Check sheet for the modelled part. Datum: model origin and axes. Units: mm. Give positions to 0.01 mm unless a question says otherwise; leave off trailing zeros. Order: outer loops, then holes, each group sorted by start corner. A loop starts at its lowest first (then second) coordinate and runs counter-clockwise, first axis right, second up.
Item 1: Sectioned sample at C-C on x = 363. Record the boundary of the cut face in (y, z).
Item 2: Sectioned sample at D-D on y = 85. Record the boundary of the cut face in (x, z), and give its area (3 significant figures).
Item 3: Sectioned sample at B-B on z = 16. Record the boundary of the cut face in (x, y), and give its area (3 significant figures).
Item 4: Material ranges on line 1 along Y through (x, z) = (-82, 11.25); line 2 along Y through (x, z) = (64.5, 5.25), recorded low to high.
Item 5: Sectioned sample at A-A on y = 49.5. Record the boundary of the cut face in (x, z), and give its area (3 significant figures).
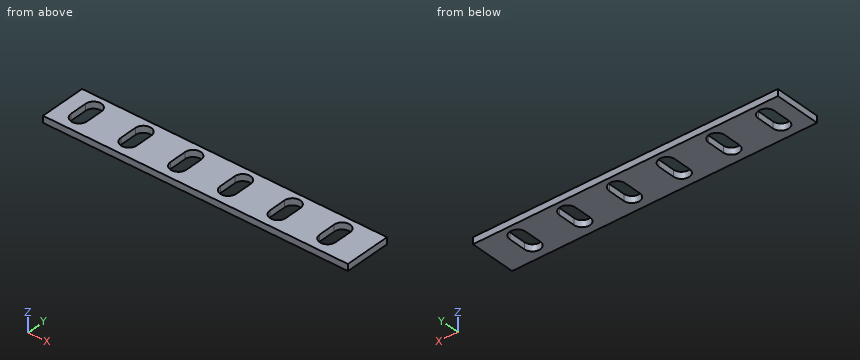
from build123d import *

# Parameters (mm, degrees)
SKETCH1_W           = 920
SKETCH1_H           = 140
BOSS_EXTRUDE1_DEPTH = 20


with BuildPart() as part:
    # Sketch1 → Boss-Extrude1 (new body)
    with BuildSketch(Plane.XY):
        with Locations((9.62605042, 42.521008403)):
            Rectangle(SKETCH1_W, SKETCH1_H)
        with BuildLine():
            Line((-358.161990974, 72.74106151), (-358.161990974, 20.74106151))
            ThreePointArc((-358.161990974, 20.74106151), (-382.161990974, -3.25893849), (-406.161990974, 20.74106151))
            Line((-406.161990974, 20.74106151), (-406.161990974, 72.74106151))
            ThreePointArc((-406.161990974, 72.74106151), (-382.161990974, 96.74106151), (-358.161990974, 72.74106151))
        make_face(mode=Mode.SUBTRACT)
        with BuildLine():
            Line((-208.161990974, 72.74106151), (-208.161990974, 20.74106151))
            ThreePointArc((-208.161990974, 20.74106151), (-232.161990974, -3.25893849), (-256.161990974, 20.74106151))
            Line((-256.161990974, 20.74106151), (-256.161990974, 72.74106151))
            ThreePointArc((-256.161990974, 72.74106151), (-232.161990974, 96.74106151), (-208.161990974, 72.74106151))
        make_face(mode=Mode.SUBTRACT)
        with BuildLine():
            Line((-58.161990974, 72.74106151), (-58.161990974, 20.74106151))
            ThreePointArc((-58.161990974, 20.74106151), (-82.161990974, -3.25893849), (-106.161990974, 20.74106151))
            Line((-106.161990974, 20.74106151), (-106.161990974, 72.74106151))
            ThreePointArc((-106.161990974, 72.74106151), (-82.161990974, 96.74106151), (-58.161990974, 72.74106151))
        make_face(mode=Mode.SUBTRACT)
        with BuildLine():
            Line((91.838009026, 72.74106151), (91.838009026, 20.74106151))
            ThreePointArc((91.838009026, 20.74106151), (67.838009026, -3.25893849), (43.838009026, 20.74106151))
            Line((43.838009026, 20.74106151), (43.838009026, 72.74106151))
            ThreePointArc((43.838009026, 72.74106151), (67.838009026, 96.74106151), (91.838009026, 72.74106151))
        make_face(mode=Mode.SUBTRACT)
        with BuildLine():
            Line((241.838009026, 72.74106151), (241.838009026, 20.74106151))
            ThreePointArc((241.838009026, 20.74106151), (217.838009026, -3.25893849), (193.838009026, 20.74106151))
            Line((193.838009026, 20.74106151), (193.838009026, 72.74106151))
            ThreePointArc((193.838009026, 72.74106151), (217.838009026, 96.74106151), (241.838009026, 72.74106151))
        make_face(mode=Mode.SUBTRACT)
        with BuildLine():
            Line((391.838009026, 72.74106151), (391.838009026, 20.74106151))
            ThreePointArc((391.838009026, 20.74106151), (367.838009026, -3.25893849), (343.838009026, 20.74106151))
            Line((343.838009026, 20.74106151), (343.838009026, 72.74106151))
            ThreePointArc((343.838009026, 72.74106151), (367.838009026, 96.74106151), (391.838009026, 72.74106151))
        make_face(mode=Mode.SUBTRACT)
    extrude(amount=BOSS_EXTRUDE1_DEPTH)


solid = part.part
Report:
1. outline: (-27.48, 0) - (-2.77, 0) - (-2.77, 20) - (-27.48, 20) - close; (96.25, 0) - (112.52, 0) - (112.52, 20) - (96.25, 20) - close
2. outline: (-450.37, 0) - (-402.79, 0) - (-402.79, 20) - (-450.37, 20) - close; (-361.53, 0) - (-252.79, 0) - (-252.79, 20) - (-361.53, 20) - close; (-211.53, 0) - (-102.79, 0) - (-102.79, 20) - (-211.53, 20) - close; (-61.53, 0) - (47.21, 0) - (47.21, 20) - (-61.53, 20) - close; (88.47, 0) - (197.21, 0) - (197.21, 20) - (88.47, 20) - close; (238.47, 0) - (347.21, 0) - (347.21, 20) - (238.47, 20) - close; (388.47, 0) - (469.63, 0) - (469.63, 20) - (388.47, 20) - close
2. area: 13,400 mm2
3. outline: (-450.37, -27.48) - (469.63, -27.48) - (469.63, 112.52) - (-450.37, 112.52) - close; hole (-406.16, 20.74) arc R24 ccw to (-358.16, 20.74) - (-358.16, 72.74) arc R24 ccw to (-406.16, 72.74) - close; hole (-256.16, 20.74) arc R24 ccw to (-208.16, 20.74) - (-208.16, 72.74) arc R24 ccw to (-256.16, 72.74) - close; hole (-106.16, 20.74) arc R24 ccw to (-58.16, 20.74) - (-58.16, 72.74) arc R24 ccw to (-106.16, 72.74) - close; hole (43.84, 20.74) arc R24 ccw to (91.84, 20.74) - (91.84, 72.74) arc R24 ccw to (43.84, 72.74) - close; hole (193.84, 20.74) arc R24 ccw to (241.84, 20.74) - (241.84, 72.74) arc R24 ccw to (193.84, 72.74) - close; hole (343.84, 20.74) arc R24 ccw to (391.84, 20.74) - (391.84, 72.74) arc R24 ccw to (343.84, 72.74) - close
3. area: 103,000 mm2
4. line 1: y = -27.48 to -3.26, 96.74 to 112.52
4. line 2: y = -27.48 to -3.03, 96.51 to 112.52
5. outline: (-450.37, 0) - (-406.16, 0) - (-406.16, 20) - (-450.37, 20) - close; (-358.16, 0) - (-256.16, 0) - (-256.16, 20) - (-358.16, 20) - close; (-208.16, 0) - (-106.16, 0) - (-106.16, 20) - (-208.16, 20) - close; (-58.16, 0) - (43.84, 0) - (43.84, 20) - (-58.16, 20) - close; (91.84, 0) - (193.84, 0) - (193.84, 20) - (91.84, 20) - close; (241.84, 0) - (343.84, 0) - (343.84, 20) - (241.84, 20) - close; (391.84, 0) - (469.63, 0) - (469.63, 20) - (391.84, 20) - close
5. area: 12,600 mm2
